Work out the finished part from the listing and answer in its coordinate system (mm). Face numbers are marked on the shaded views. A direction names the side the tool comes from. Coordinates: 2 decimals unless noted, no trailing zeros. Order: outer loops, then holes, each group sorted by start corner. A loop starts at its lowest first (then second) coordinate and runs counter-clockwise, first axis right, second up. Notation, with made-up numbers: M -1.5,60 L 31.5,60 A11 ccw 31.5,68 Z; hole C 11.25,-40 d4. An arc over 180 degrees is marked long. Answer in a Markdown table with one row per item. Add a question column.
Item 1: The part is cut by section D-D (z = 13). Write down the section's boundary in (x, y), then the cut area to 3 significant figures.
Item 2: Which of the six approach directions +Z, -Z, +X, -X, +Y, -Y give full straight-line access (tool end or side, diameter ignored) to the marked faces 4 and 5?
Item 3: The part is cut by section A-A (x = 0). Write down the section's boundary in (y, z).
Item 4: The part is cut by section C-C (z = 2.5). Write down the section's boundary in (x, y).
Item 5: Flat-ended cylindrical pins translate along their axes: pin 1 Ø1.5 at (y, z) = (5, 26.5) entering from -X; pin 2 Ø4 at (x, z) = (-21.5, 3.5) entering from +Y; pin 3 Ø3 at (x, y) = (-20, 13.5) entering from +Z. Find the tip coordinate at first contact, or state that the pin passes through.
Item 6: The mould has two halves that part along X. Classify the marked faces 1, 2 and 3: released by +X, released by -X, zero draft, split by the parting line, or undercut.
Item 7: The part is cut by section B-B (y = 0). Write down the section's boundary in (x, z).
Item 8: Consider line 1 (Z direction, x = -9.5, y = 9); line 2 (X direction, y = 6, z = 2); line 3 (Z direction, x = 2, y = -27.5). Determine where each line is inside the solid, lowest interval first. Write a range as from..to.
from build123d import *

# Parameters (mm, degrees)
F0_R     = 30
F1_DEPTH = 14
F2_R     = 24
F3_DEPTH = 20
F4_SIZE  = 1.5
F6_DEPTH = 1.5
F8_D     = 4.2
F8_DEPTH = 10
F8_TIP   = 1.2618073


with BuildPart() as f1:
    # F0 (on Top) → F1 (new body)
    with BuildSketch(Plane.XY):
        Circle(F0_R)
    extrude(amount=F1_DEPTH)

    # F2 (on face) → F3 (join)
    with BuildSketch(Plane.XY.offset(14)):
        Circle(F2_R)
    extrude(amount=F3_DEPTH)

    # F4
    f4_edges = [f1.edges().sort_by_distance(p)[0] for p in [
        (-24, 0, 34),
    ]]
    chamfer(f4_edges, length=F4_SIZE)

    # F5 (on face) → F6 (cut)
    with BuildSketch(Plane(origin=(0, 0, 0), x_dir=(1, 0, 0), z_dir=(0, 0, -1))):
        with BuildLine():
            Line((18, 36.3252682028), (-18, 36.3252682028))
            Line((-18, 36.3252682028), (-18, 24))
            ThreePointArc((-18, 24), (0, 30), (18, 24))
            Line((18, 24), (18, 36.3252682028))
        make_face()
        with BuildLine():
            ThreePointArc((18, 24), (0, 30), (-18, 24))
            Line((-18, 24), (-18, -24))
            ThreePointArc((-18, -24), (0, -30), (18, -24))
            Line((18, -24), (18, 24))
        make_face()
        with BuildLine():
            ThreePointArc((18, -24), (0, -30), (-18, -24))
            Line((-18, -24), (-18, -38.8747264979))
            Line((-18, -38.8747264979), (18, -38.8747264979))
            Line((18, -38.8747264979), (18, -24))
        make_face()
    extrude(amount=-F6_DEPTH, mode=Mode.SUBTRACT)

    # F8
    with Locations(Plane(origin=(0, 0, 0), x_dir=(1, 0, 0), z_dir=(0, 0, -1))):
        with Locations((-24.1402154091, 6.5), (24.1402154091, -6.5)):
            Hole(F8_D / 2, depth=F8_DEPTH)
            with Locations((0, 0, -(F8_DEPTH + F8_TIP / 2))):  # 118° drill point
                Cone(0, F8_D / 2, F8_TIP, mode=Mode.SUBTRACT)


solid = f1.part
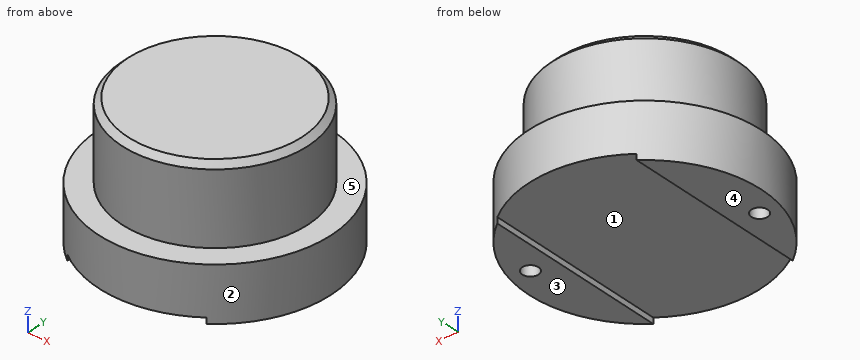
Reply:
| question | item | result |
|---|---|---|
| 1 | outline | C 0,0 d60 |
| 1 | area | 2,830 mm2 |
| 2 | face 4 | -Z, +X, -X, +Y, -Y |
| 2 | face 5 | +Z |
| 3 | outline | M -30,1.5 L 30,1.5 L 30,14 L 24,14 L 24,32.5 L 22.5,34 L -22.5,34 L -24,32.5 L -24,14 L -30,14 Z |
| 4 | outline | C 0,0 d60; hole C -24.14,-6.5 d4.2; hole C 24.14,6.5 d4.2 |
| 5 | pin 1 | stops at x = -23.62 |
| 5 | pin 2 | stops at y = 22.8 |
| 5 | pin 3 | stops at z = 33.87 |
| 6 | face 1 | undercut |
| 6 | face 2 | split by the parting line |
| 6 | face 3 | zero draft |
| 7 | outline | M -30,0 L -18,0 L -18,1.5 L 18,1.5 L 18,0 L 30,0 L 30,14 L 24,14 L 24,32.5 L 22.5,34 L -22.5,34 L -24,32.5 L -24,14 L -30,14 Z |
| 8 | line 1 | z = 1.5..34 |
| 8 | line 2 | x = -29.39..22.1, 26.18..29.39 |
| 8 | line 3 | z = 1.5..14 |
